Build history of the part. All positions in model axes, mm. A direction names the side the tool comes from. Give positions to 0.01 mm unless a question says otherwise; leave off trailing zeros. Loops run counter-clockwise (first coordinate to the right, second up) from the corner with the lowest first, then second, coordinate; pieces in that order, holes last. Notation, with made-up numbers: (75.25, 55) -> (134.25, 55) arc R14 cw to (134.25, 64) -> close; hole circle Ø2 at (-2, 3). An arc over 180 degrees is marked (long way). Answer as a JSON object with one key per item and string values. Group by question number.
Q1. Two-plate mould, pull along Y, no slides. Class faces 1 (the flat face through (10, 0, 0)), 2 (the flat face through (19.72, -2.39, -1.36)), 3 (the flat face through (19.721, 2.37, -1.394)): pulls with the +Y half, pulls with the -Y half, needs draft (parallel to the pull), parting line crosses it, or undercut.
Q2. Band-saw the part on B-B, the plane y = 0. Write the cut outline in (x, z).
Q3. Wall check: probe 1 along Y at (x, z) = (4, 0); probe 2 along X at (y, z) = (-1.5, -1.6); probe 3 along X at (y, z) = (0.5, 0.8). Give the ranges that are in metal, low to high. Write a range as from..to.
Q4. Drop a flat-ended pin along its axis: pin 1 (0.9 mm diameter, centred on y = 0.5, z = -0.5, fed in from -X). Give the stop position or say it passes through.
Q5. Band-saw the part on D-D, the plane x = 44. Write the cut outline in (y, z), plus the area to 3 significant figures.
Q6. Band-saw the part on C-C, the plane x = 32. Write the cut outline in (y, z).
Q7. Tool access for faces 4 (the flat face through (40, -2, 0)), 5 (the cylindrical face through (4.93, 0.07, -1.5)), 6 (the flat face through (20, 0, -2.75)): list every direction of +Z, -Z, +X, -X, +Y, -Y with a clear straight run to the whole face (end or side of a thin tool).
Q8. Band-saw the part on A-A, the plane x = 8.5. Write the cut outline in (y, z).
from build123d import *

# Parameters (mm, degrees)
BOSS_EXTRUDE1_DEPTH = 40
SKETCH2_R           = 1.5
BOSS_EXTRUDE2_DEPTH = 8
SKETCH3_R           = 1.5
CUT_EXTRUDE1_DEPTH  = 10
CHAMFER1_SIZE       = 0.3


with BuildPart() as part:
    # Sketch1 → Boss-Extrude1 (new body)
    with BuildSketch(Plane(origin=(0, 0, 0), x_dir=(0, 0, -1), z_dir=(1, 0, 0))):
        Polygon((0, 3.175426481), (-2.75, 1.58771324), (-2.75, -1.58771324), (0, -3.175426481), (2.75, -1.58771324), (2.75, 1.58771324), align=None)
    extrude(amount=BOSS_EXTRUDE1_DEPTH)

    # Sketch2 → Boss-Extrude2 (add)
    with BuildSketch(Plane(origin=(40, 0, 0), x_dir=(0, 0, -1), z_dir=(1, 0, 0))):
        Circle(SKETCH2_R)
    extrude(amount=BOSS_EXTRUDE2_DEPTH)

    # Sketch3 → Cut-Extrude1 (cut)
    with BuildSketch(Plane.ZY):
        Circle(SKETCH3_R)
    extrude(amount=-CUT_EXTRUDE1_DEPTH, mode=Mode.SUBTRACT)

    # Sketch4 → Cut-Revolve1 (revolve, cut)
    with BuildSketch(Plane(origin=(0, 0, 0), x_dir=(1, 0, 0), z_dir=(0, 1, 0))):
        Polygon((0, 10.219809024), (4.392081913, 10.219809024), (0, 2.6125), align=None)
        Polygon((40, 2.6125), (40, 10.219809024), (35.607918087, 10.219809024), align=None)
    revolve(axis=Axis((0, 0, 0), (-1, 0, 0)), mode=Mode.SUBTRACT)

    # Chamfer1
    chamfer1_edges = [part.edges().sort_by_distance(p)[0] for p in [
        (48, 0, 1.5),
    ]]
    chamfer(chamfer1_edges, length=CHAMFER1_SIZE)


solid = part.part
Worked answers:
{
 "1": {"face 1": "undercut", "face 2": "pulls with the -Y half", "face 3": "pulls with the +Y half"},
 "2": {"outline": "(0, -2.61) -> (0.08, -2.75) -> (39.92, -2.75) -> (40, -2.61) -> (40, -1.5) -> (47.7, -1.5) -> (48, -1.2) -> (48, 1.2) -> (47.7, 1.5) -> (40, 1.5) -> (40, 2.61) -> (39.92, 2.75) -> (0.08, 2.75) -> (0, 2.61) -> (0, 1.5) -> (10, 1.5) -> (10, -1.5) -> (0, -1.5) -> close"},
 "3": {"probe 1": "-3.18..-1.5, 1.5..3.18", "probe 2": "0..40", "probe 3": "10..48"},
 "4": {"pin 1": "x = 10"},
 "5": {"outline": "circle Ø3 at (0, 0)", "area": "7.07 mm2"},
 "6": {"outline": "(-3.18, 0) -> (-1.59, -2.75) -> (1.59, -2.75) -> (3.18, 0) -> (1.59, 2.75) -> (-1.59, 2.75) -> close"},
 "7": {"face 4": "+X", "face 5": "-X", "face 6": "-Z, +X, -X, +Y, -Y"},
 "8": {"outline": "(-3.18, 0) -> (-1.59, -2.75) -> (1.59, -2.75) -> (3.18, 0) -> (1.59, 2.75) -> (-1.59, 2.75) -> close; hole circle Ø3 at (0, 0)"}
}
